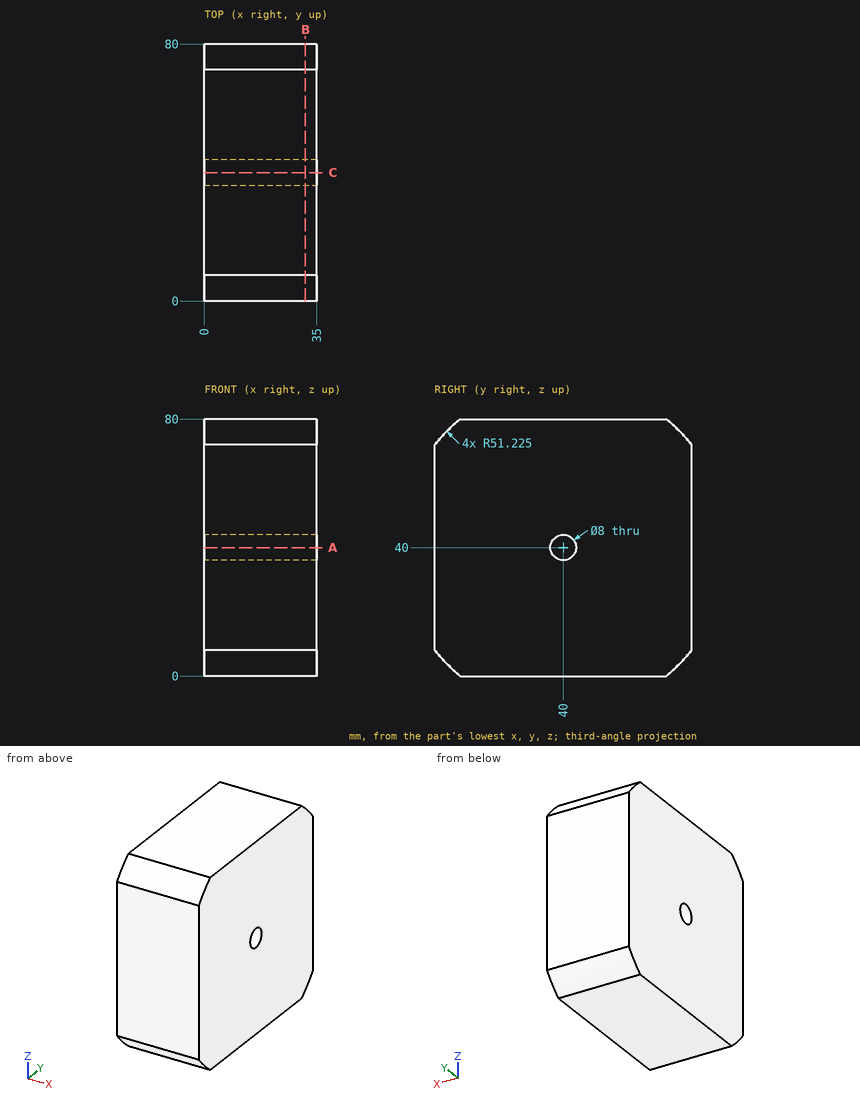
Answer from the drawing. Dimensions are ordinates in mm from the lowest x, y and z of the part. Give positions to 0.01 mm unless a question says otherwise; leave off trailing zeros. Write each loop counter-clockwise with the first axis right and the second up, starting at its lowest first coordinate (ties: lowest second). Pieces come first, ordered by that corner, then holes. Notation, with made-up numbers: (3, 3.5) - (33, 3.5) arc R18 ccw to (33, 31.5) - close; hole circle Ø4 at (59, 78). An arc over 180 degrees is marked (long way). Answer in a Markdown table with one row per item. Add a question column.
Item 1: Find the intervals of material crossed by L1, parallel to Z at x = 12, y = 40; L2, parallel to Z at x = 9, y = 37; L3, parallel to Y at x = 33, z = 43.5, in increasing order.
Item 2: Section A-A, the plane z = 40 is taken. Write down the section's boundary in (x, y).
Item 3: Section B-B, the plane x = 31.5 is taken. Write down the section's boundary in (y, z) (3 decimals), and give its area (3 significant figures).
Recorded:
| question | item | result |
|---|---|---|
| 1 | L1 | z = 0 to 36, 44 to 80 |
| 1 | L2 | z = 0 to 37.35, 42.65 to 80 |
| 1 | L3 | y = 0 to 38.06, 41.94 to 80 |
| 2 | outline | (0, 0) - (35, 0) - (35, 36) - (0, 36) - close; (0, 44) - (35, 44) - (35, 80) - (0, 80) - close |
| 3 | outline | (0, 8) arc R51.225 ccw to (8, 0) - (72, 0) arc R51.225 ccw to (80, 8) - (80, 72) arc R51.225 ccw to (72, 80) - (8, 80) arc R51.225 ccw to (0, 72) - close; hole circle Ø8 at (40, 40) |
| 3 | area | 6,230 mm2 |
